Part model, mm, in its own coordinate system. A direction names the side the tool comes from. Give positions to 0.01 mm unless a question says otherwise; leave off trailing zeros. Loops run counter-clockwise (first coordinate to the right, second up) from the corner with the lowest first, then second, coordinate; pieces in that order, holes last. Notation, with made-up numbers: M 72.5,66 L 94.5,66 A23 ccw 94.5,104 Z; hole C -11,32 d11. An arc over 180 degrees is marked long. Answer in a Markdown table with one row per item.
from build123d import *

# Parameters (mm, degrees)
SKETCH1_W           = 114
SKETCH1_H           = 104
BOSS_EXTRUDE1_DEPTH = 3
SKETCH2_W           = 114
SKETCH2_H           = 104
SKETCH2_W_2         = 110
SKETCH2_H_2         = 100
BOSS_EXTRUDE2_DEPTH = 50
SKETCH3_W           = 5
SKETCH3_H           = 5
BOSS_EXTRUDE4_DEPTH = 7
SKETCH8_W           = 114
SKETCH8_H           = 53
BOSS_EXTRUDE6_DEPTH = 5
SKETCH9_W           = 110
SKETCH9_H           = 50
CUT_EXTRUDE2_DEPTH  = 5
SKETCH12_W          = 8
SKETCH12_H          = 10
CUT_EXTRUDE3_DEPTH  = 2
SKETCH14_R          = 1
CUT_EXTRUDE5_DEPTH  = 3
SKETCH15_R          = 2
CUT_EXTRUDE6_DEPTH  = 3


with BuildPart() as part:
    # Sketch1 → Boss-Extrude1 (new body)
    with BuildSketch(Plane(origin=(0, 0, 0), x_dir=(1, 0, 0), z_dir=(0, 1, 0))):
        Rectangle(SKETCH1_W, SKETCH1_H)
    extrude(amount=BOSS_EXTRUDE1_DEPTH)

    # Sketch2 → Boss-Extrude2 (add)
    with BuildSketch(Plane(origin=(0, 3, 0), x_dir=(1, 0, 0), z_dir=(0, 1, 0))):
        Rectangle(SKETCH2_W, SKETCH2_H)
        Rectangle(SKETCH2_W_2, SKETCH2_H_2, mode=Mode.SUBTRACT)
    extrude(amount=BOSS_EXTRUDE2_DEPTH)

    # Sketch3 → Boss-Extrude4 (add)
    with BuildSketch(Plane(origin=(0, 3, 0), x_dir=(1, 0, 0), z_dir=(0, 1, 0))):
        with Locations((-6.5, 41.5)):
            Rectangle(SKETCH3_W, SKETCH3_H)
        with Locations((52.5, 46.5)):
            Rectangle(SKETCH3_W, SKETCH3_H)
        with Locations((-6.5, -41.5)):
            Rectangle(SKETCH3_W, SKETCH3_H)
        with Locations((37.5, -41.5)):
            Rectangle(SKETCH3_W, SKETCH3_H)
    extrude(amount=BOSS_EXTRUDE4_DEPTH)

    # Sketch8 → Boss-Extrude6 (add)
    with BuildSketch(Plane.XY.offset(52)):
        with Locations((0, 26.5)):
            Rectangle(SKETCH8_W, SKETCH8_H)
    extrude(amount=BOSS_EXTRUDE6_DEPTH)

    # Sketch9 → Cut-Extrude2 (cut)
    with BuildSketch(Plane(origin=(0, 0, 50), x_dir=(-1, 0, 0), z_dir=(0, 0, -1))):
        with Locations((0, 28)):
            Rectangle(SKETCH9_W, SKETCH9_H)
    extrude(amount=-CUT_EXTRUDE2_DEPTH, mode=Mode.SUBTRACT)

    # Sketch12 → Cut-Extrude3 (cut)
    with BuildSketch(Plane(origin=(-55, 0, 0), x_dir=(0, 0, -1), z_dir=(1, 0, 0))):
        with Locations((-3, 8)):
            Rectangle(SKETCH12_W, SKETCH12_H)
    extrude(amount=-CUT_EXTRUDE3_DEPTH, mode=Mode.SUBTRACT)

    # Sketch14 → Cut-Extrude5 (cut)
    with BuildSketch(Plane(origin=(0, 10, 0), x_dir=(1, 0, 0), z_dir=(0, 1, 0))):
        with Locations((-6.5, 41.5)):
            Circle(SKETCH14_R)
        with Locations((-6.5, -41.5)):
            Circle(SKETCH14_R)
        with Locations((37.5, -41.5)):
            Circle(SKETCH14_R)
        with Locations((52.5, 46.5)):
            Circle(SKETCH14_R)
    extrude(amount=-CUT_EXTRUDE5_DEPTH, mode=Mode.SUBTRACT)

    # Sketch15 → Cut-Extrude6 (cut)
    with BuildSketch(Plane(origin=(0, 3, 0), x_dir=(1, 0, 0), z_dir=(0, 1, 0))):
        with Locations((-50, 45)):
            Circle(SKETCH15_R)
        with Locations((-50, -50)):
            Circle(SKETCH15_R)
        with Locations((43.810047303, -50)):
            Circle(SKETCH15_R)
        with Locations((43.810047303, 45)):
            Circle(SKETCH15_R)
    extrude(amount=-CUT_EXTRUDE6_DEPTH, mode=Mode.SUBTRACT)


solid = part.part
(1) Drill centre lines: line 1 along X through (y, z) = (8.95, -46.5); line 2 along Z through (x, y) = (-50, 2.2); line 3 along Z through (x, y) = (52.5, 8.1). Where is each one in solid material? Low to high.
Recorded:
| item | result |
|---|---|
| line 1 | x = -57 to -55, 50 to 51.5, 53.5 to 57 |
| line 2 | z = -52 to -47, -43 to 48, 52 to 57 |
| line 3 | z = -52 to -50, -49 to -47.5, -45.5 to -44, 55 to 57 |
(2) Saw through at C-C (z = 50). Write the cut outline in (x, y), plus the area to 3 significant figures.
Recorded:
| item | result |
|---|---|
| outline | M -57,0 L -52,0 L -52,3 L -55,3 L -55,53 L -57,53 Z; M -48,0 L 41.81,0 L 41.81,3 L -48,3 Z; M 45.81,0 L 57,0 L 57,53 L 55,53 L 55,3 L 45.81,3 Z |
| area | 518 mm^2 |
(3) Pin check, flat tips, straight feed: pin 1 Ø4 at (x, z) = (51.5, -46.5) entering from +Y; pin 2 Ø3 at (x, z) = (52.5, -46.5) entering from -Y; pin 3 Ø1.2 at (x, z) = (-6.5, -41.5) entering from +Y; pin 4 Ø2 at (y, z) = (9.5, 0.5) entering from -X. Stop position of each tip, or through.
Recorded:
| item | result |
|---|---|
| pin 1 | stops at y = 10 |
| pin 2 | stops at y = 0 |
| pin 3 | stops at y = 7 |
| pin 4 | stops at x = 55 |
(4) Saw through at B-B (x = -50). Write the cut outline in (y, z), plus the area to 3 significant figures.
Recorded:
| item | result |
|---|---|
| outline | M 0,-52 L 53,-52 L 53,-50 L 3,-50 L 3,-47 L 0,-47 Z; M 0,-43 L 3,-43 L 3,48 L 0,48 Z; M 0,52 L 3,52 L 3,55 L 53,55 L 53,57 L 0,57 Z |
| area | 503 mm^2 |
(5) Saw through at D-D (y = 15). Write the cut outline in (x, z).
Recorded:
| item | result |
|---|---|
| outline | M -57,-52 L 57,-52 L 57,57 L -57,57 Z; hole M -55,-50 L 55,-50 L 55,55 L -55,55 Z |
(6) Saw through at A-A (z = 4). Write the cut outline in (x, y).
Recorded:
| item | result |
|---|---|
| outline | M -57,0 L 57,0 L 57,53 L 55,53 L 55,3 L -57,3 Z; M -57,13 L -55,13 L -55,53 L -57,53 Z |
(7) Pull direction X, two halves, no side cores. Call faces 1 (the face through (37, 6, 44)), 2 (the face through (57, 26, 2)), 3 (the face through (-1, 0, 2)): +X half, -X half, draft (parallel to the pull), parting line (faces both ways), or undercut.
Recorded:
| item | result |
|---|---|
| face 1 | undercut |
| face 2 | +X half |
| face 3 | draft |
(8) Which spindle directions (+Z, -Z, +X, -X, +Y, -Y) get a long thin tool onto all of the face, cutting with end or side? Do faces 4 (the face through (-1, 26, -52)), 5 (the face through (40, 6, 42)). Say none if no direction does.
Recorded:
| item | result |
|---|---|
| face 4 | -Z, +X, -X, +Y, -Y |
| face 5 | +Y |
